CAD build for the part. Positions are in the model's coordinates, mm. Face numbers are marked on the shaded views. A direction names the side the tool comes from. Give positions to 0.01 mm unless a question says otherwise; leave off trailing zeros. Write each loop counter-clockwise with the first axis right and the second up, starting at its lowest first coordinate (ties: lowest second). Pieces come first, ordered by that corner, then holes. Notation, with made-up numbers: (-28.75, 58) - (-22.75, 58) arc R31 cw to (-22.75, 88) - close; hole circle Ø3 at (49.25, 63.25). An arc over 180 degrees is marked (long way). Put each result on its own line as item: value. Start each with the question number.
1. Cut at B-B on z = -5.5. List the corners of the cut face in (x, y), and give its area (3 significant figures).
2. Cut at D-D on x = 14.4. List the corners of the cut face in (y, z), and give its area (3 significant figures).
3. Drop flat-ended pins along their axis: pin 1 (1 mm diameter, centred on x = 98, y = -34, fed in from +Z); pin 2 (3 mm diameter, centred on x = 99, z = 12, fed in from -Y); pin 3 (0.6 mm diameter, centred on x = 57, y = -46, fed in from +Z). Give the stop position or say it passes through.
4. Mould opens along X. For the marked faces 1, 2 and 3 say: +X half, -X half, draft (parallel to the pull), parting line (faces both ways), or undercut.
5. Cut at A-A on x = 98.1. List the corners of the cut face in (y, z).
6. Tool access for the marked faces 4 and 5: list every direction of +Z, -Z, +X, -X, +Y, -Y with a clear straight run to the whole face (end or side of a thin tool).
7. Wall check: line 1 (Y direction, x = 55.5, z = 4); line 2 (X direction, y = -6, z = -43.5); line 3 (Y direction, x = 51.5, z = -39). Give the ranges that are in metal, low to high.
8. Cut at C-C on y = -3.5. List the corners of the cut face in (x, z).
from build123d import *

# Parameters (mm, degrees)
F1_DEPTH  = 115
F3_START  = -2
F2_W      = 111
F2_H      = 50.45
F3_DEPTH  = 173.4
F4_W      = 47.4
F4_H      = 28.25
F4_R      = 1
F5_DEPTH  = 25
F7_DEPTH  = 2
F8_R      = 2.5
F9_DEPTH  = 5.7
F10_R     = 2
F11_DEPTH = 25
F12_R     = 5
F14_DEPTH = 8.7
F15_R     = 10


with BuildPart() as f1:
    # F0 (on Right) → F1 (new body)
    with BuildSketch(Plane.YZ):
        Polygon((-46.95, 9.6120529463), (-46.95, -64.3379470537), (7, -64.3379470537), (7, 30.95759285), (7, 58.6620529463), (0, 58.6620529463), align=None)
    extrude(amount=F1_DEPTH)

    # F2 (on face) → F3 (cut)
    with BuildSketch(Plane(origin=(0, 0, -64.3379470537), x_dir=(1, 0, 0), z_dir=(0, 0, -1)).offset(F3_START)):
        with Locations((57.5, 19.725)):
            Rectangle(F2_W, F2_H)
    extrude(amount=-F3_DEPTH, mode=Mode.SUBTRACT)

    # F4 (on face) → F5 (cut)
    with BuildSketch(Plane.XZ.offset(46.95)):
        with Locations((57.5, -39.2129470537)):
            Rectangle(F4_W, F4_H)
        with Locations((57.75, -19.4129470537)):
            Circle(F4_R)
        with Locations((57.75, -59.0129470537)):
            Circle(F4_R)
    extrude(amount=-F5_DEPTH, mode=Mode.SUBTRACT)

    # F6 (on face) → F7 (cut)
    with BuildSketch(Plane(origin=(0, 7, 0), x_dir=(-1, 0, 0), z_dir=(0, 1, 0))):
        with BuildLine():
            Line((-36.4904825576, -54.8379470537), (-36.4904825576, -62.3379470537))
            Line((-36.4904825576, -62.3379470537), (-11.4904825576, -62.3379470537))
            Line((-11.4904825576, -62.3379470537), (-11.4904825576, -54.8379470537))
            ThreePointArc((-11.4904825576, -54.8379470537), (-23.9904825576, -42.3379470537), (-36.4904825576, -54.8379470537))
        make_face()
    extrude(amount=-F7_DEPTH, mode=Mode.SUBTRACT)

    # F8 (on face) → F9 (cut)
    with BuildSketch(Plane(origin=(0, 7, 0), x_dir=(-1, 0, 0), z_dir=(0, 1, 0))):
        with Locations((-98.1, 43.6620529463)):
            Circle(F8_R)
        with Locations((-14.4, 43.6620529463)):
            Circle(F8_R)
    extrude(amount=-F9_DEPTH, mode=Mode.SUBTRACT)

    # F10 (on face) → F11 (cut)
    with BuildSketch(Plane.YZ.offset(115)):
        with Locations((-20.65, 4.6679739505)):
            Circle(F10_R)
    extrude(amount=-F11_DEPTH, mode=Mode.SUBTRACT)

    # F12
    f12_edges = [f1.edges().sort_by_distance(p)[0] for p in [
        (1, 0, 58.662053),
        (114, 0, 58.662053),
    ]]
    fillet(f12_edges, radius=F12_R)

    # F13 (on face) → F14 (cut)
    with BuildSketch(Plane(origin=(0, 0, -64.3379470537), x_dir=(1, 0, 0), z_dir=(0, 0, -1))):
        with BuildLine():
            Line((11.490044184, 3.5827266984), (11.490044184, -7))
            Line((11.490044184, -7), (36.4903211594, -7))
            Line((36.4903211594, -7), (36.4903211594, 3.5827266984))
            ThreePointArc((36.4903211594, 3.5827266984), (23.9901826717, 9.3848176292), (11.490044184, 3.5827266984))
        make_face()
    extrude(amount=-F14_DEPTH, mode=Mode.SUBTRACT)

    # F15
    f15_edges = [f1.edges().sort_by_distance(p)[0] for p in [
        (36.490321, -3.582727, -63.337947),
        (11.490044, -3.582727, -63.337947),
    ]]
    fillet(f15_edges, radius=F15_R)


solid = f1.part
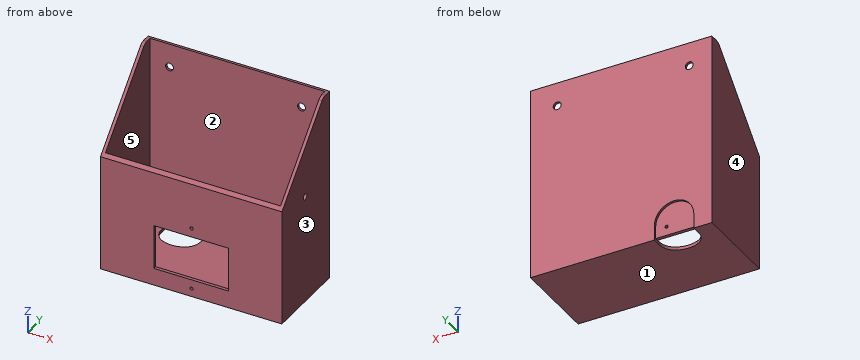
Report:
1. outline: (0, -46.95) - (115, -46.95) - (115, 7) - (0, 7) - close; hole (2, -44.95) - (113, -44.95) - (113, 5.5) - (2, 5.5) - close
1. area: 604 mm²
2. outline: (-46.95, -64.34) - (-5.93, -64.34) - (-5.93, -62.34) - (-44.95, -62.34) - (-44.95, 11.7) - (-46.95, 9.61) - close; (5.5, -46.82) - (7, -46.82) - (7, 41.16) - (5.5, 41.16) - close; (5.5, 46.16) - (7, 46.16) - (7, 58.66) - (5.5, 58.66) - close
2. area: 379 mm²
3. pin 1: stops at z = -62.34
3. pin 2: stops at y = -46.1
3. pin 3: stops at z = 10.92
4. face 1: draft
4. face 2: undercut
4. face 3: +X half
5. outline: (-46.95, -64.34) - (7, -64.34) - (7, 41.16) - (5.5, 41.16) - (5.5, -62.34) - (-44.95, -62.34) - (-44.95, 11.7) - (-46.95, 9.61) - close; (5.5, 46.16) - (7, 46.16) - (7, 58.66) - (5.5, 58.66) - close
6. face 4: +Z, -Z, -X, +Y, -Y
6. face 5: +Z
7. line 1: y = -46.95 to -44.95, 5.5 to 7
7. line 2: x = 0 to 2, 113 to 115
7. line 3: y = 5.5 to 7
8. outline: (0, -64.34) - (12.62, -64.34) - (12.62, -62.34) - (2, -62.34) - (2, 55.01) - (0, 55.01) - close; (35.36, -64.34) - (115, -64.34) - (115, 55.01) - (113, 55.01) - (113, -62.34) - (35.36, -62.34) - close
